Input: dimensioned drawing with shaded views. Units: mm. Origin: part minimum x, y, z. A direction names the side the tool comes from. Coordinates: 2 decimals unless noted, no trailing zeros. Loops run counter-clockwise (first coordinate to the right, second up) from the corner with the lowest first, then second, coordinate; pieces in that order, holes last. Notation, with made-up numbers: (82.5, 57.5) - (88.5, 57.5) arc R10 ccw to (88.5, 72.5) - close; hole circle Ø8 at (-18, -24.75). An arc over 180 degrees is marked (long way). Put each result on its own line as item: value. Start each with the question number.
1) Reachability of the marked faces 1, 2, 3 and 4 from +Z, -Z, +X, -X, +Y, -Y: full face, straight path, thin tool, end or side. Return the list, or none.
2) Section C-C on z = 50. Output: boundary loops of the cut face in (x, y).
3) Contact query for flat-ended pins moving along their axis: pin 1 Ø5 at (x, y) = (41.5, 78) entering from +Z; pin 2 Ø5 at (x, y) = (36.5, 67.5) entering from -Z; pin 3 Ø8 at (x, z) = (25, 59.5) entering from +Y. Output: stop coordinate, or through.
4) Material intervals for line 1 along Y through (x, z) = (44.5, 26); line 2 along Y through (x, z) = (37, 12); line 3 along Z through (x, y) = (9, 57), sorted ascending. Write a range as from..to.
5) Draft query along Y for the marked faces 5, 6 and 7. Return one class per face: +Y half, -Y half, draft (parallel to the pull), parting line (faces both ways), or undercut.
6) Section A-A on z = 14.5. Output: boundary loops of the cut face in (x, y), and give its area (3 significant figures).
7) Section D-D on y = 24.5. Output: boundary loops of the cut face in (x, z).
8) Section B-B on x = 4. Output: boundary loops of the cut face in (y, z).
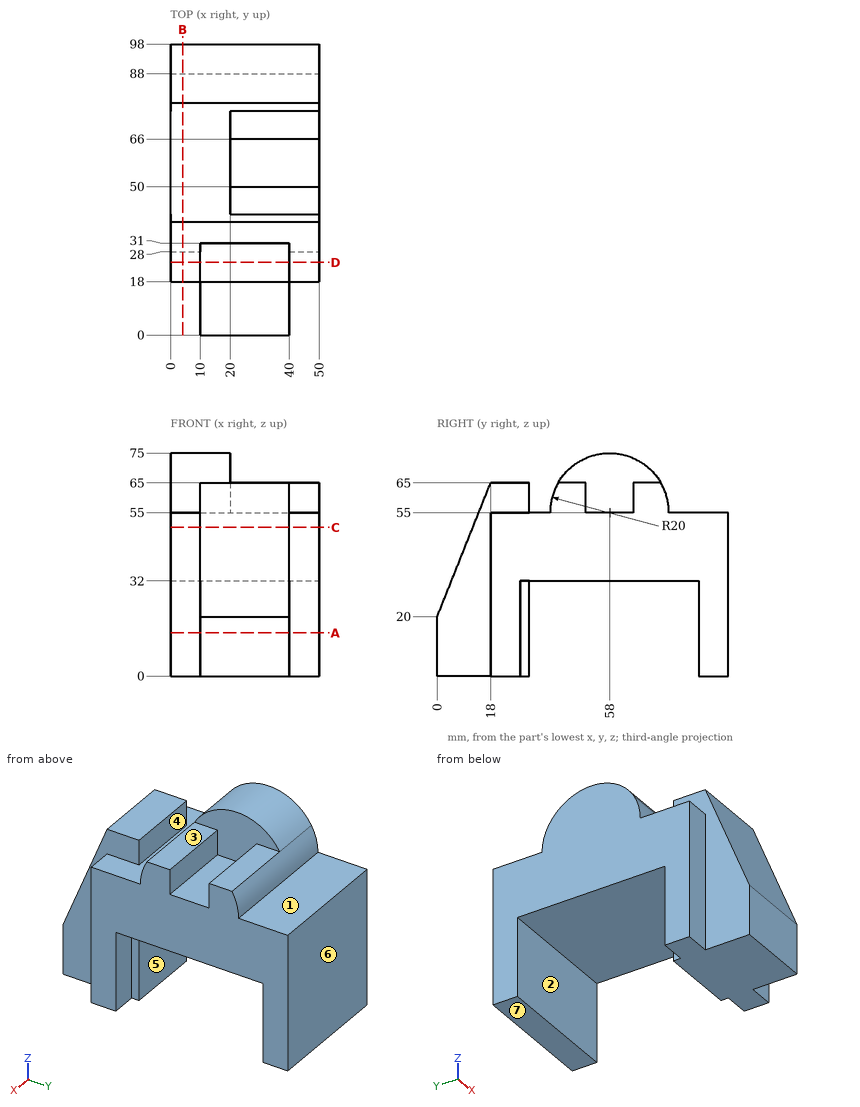
Answer block:
1. face 1: +Z, +X, -X, +Y
1. face 2: -Z, +X, -X
1. face 3: +Z, +X, +Y, -Y
1. face 4: +Z, +X, -X
2. outline: (0, 18) - (10, 18) - (10, 12) - (40, 12) - (40, 18) - (50, 18) - (50, 98) - (0, 98) - close
3. pin 1: stops at z = 64.68
3. pin 2: stops at z = 32
3. pin 3: stops at y = 77.99
4. line 1: y = 18..28, 88..98
4. line 2: y = 0..31, 88..98
4. line 3: z = 32..74.97
5. face 5: undercut
5. face 6: +Y half
5. face 7: draft
6. outline: (0, 18) - (10, 18) - (10, 0) - (40, 0) - (40, 18) - (50, 18) - (50, 28) - (40, 28) - (40, 31) - (10, 31) - (10, 28) - (0, 28) - close; (0, 88) - (50, 88) - (50, 98) - (0, 98) - close
6. area: 1,630 mm²
7. outline: (0, 0) - (50, 0) - (50, 55) - (40, 55) - (40, 65) - (10, 65) - (10, 55) - (0, 55) - close
8. outline: (18, 0) - (28, 0) - (28, 32) - (88, 32) - (88, 0) - (98, 0) - (98, 55) - (78, 55) arc R20 ccw to (38, 55) - (18, 55) - close
